Autodesk Inventor part; units mm, degrees
ref_plane "YZ Plane" through (0, 0, 0) normal (1, 0, 0) x (0, 1, 0)
ref_plane "XZ Plane" through (0, 0, 0) normal (0, 1, 0) x (-1, 0, 0)
ref_plane "XY Plane" through (0, 0, 0) normal (0, 0, 1) x (1, 0, 0)
sketch "草图7" plane through (0, 0, 0) normal (0, 1, 0) x (-1, 0, 0)
  line L0 (125, 235) -> (-125, 235)
  line L1 (-125, 235) -> (-125, -235)
  line L2 (-125, -235) -> (125, -235)
  line L3 (125, -235) -> (125, 235)
  line L4 (0, 3) -> (0, -5)
  line L5 (3.5058, 0) -> (-3.4421, 0)
  line L6 (25, 144) -> (-32, 144)
  line L7 (-32, 144) -> (-32, 87)
  line L8 (-32, 87) -> (25, 87)
  line L9 (25, 87) -> (25, 144)
  line L10 (25, 67) -> (-32, 67)
  line L11 (-32, 67) -> (-32, 10)
  line L12 (-32, 10) -> (25, 10)
  line L13 (25, 10) -> (25, 67)
  line L14 (25, -10) -> (-32, -10)
  line L15 (-32, -10) -> (-32, -67)
  line L16 (-32, -67) -> (25, -67)
  line L17 (25, -67) -> (25, -10)
  line L18 (25, -87) -> (-32, -87)
  line L19 (-32, -87) -> (-32, -144)
  line L20 (-32, -144) -> (25, -144)
  line L21 (25, -144) -> (25, -87)
  line L22 (-66, 100) -> (-95, 100)
  line L23 (-95, 100) -> (-95, 54)
  line L24 (-95, 54) -> (-66, 54)
  line L25 (-66, 54) -> (-66, 100)
  line L26 (-66, -54) -> (-95, -54)
  line L27 (-95, -54) -> (-95, -100)
  line L28 (-95, -100) -> (-66, -100)
  line L29 (-66, -100) -> (-66, -54)
  line L30 (100, 15) -> (70, 15)
  line L31 (70, 15) -> (70, -15)
  line L32 (70, -15) -> (100, -15)
  line L33 (100, -15) -> (100, 15)
  circle A0 centre (65, 182) radius 10
  circle A1 centre (65, -182) radius 10
  circle A2 centre (65, 182) radius 15
  circle A3 centre (80, 182) radius 1.5
  circle A4 centre (57.5, 194.9904) radius 1.5
  circle A5 centre (57.5, 169.0096) radius 1.5
  line L34 (125, 235) -> (0, 235)
  line L35 (0, 235) -> (0, 0)
  line L36 (0, 0) -> (125, 0)
  line L37 (125, 0) -> (125, 235)
  line L38 (-125, 235) -> (0, 235)
  line L39 (0, 235) -> (0, 0)
  line L40 (0, 0) -> (-125, 0)
  line L41 (-125, 0) -> (-125, 235)
  line L42 (-125, -235) -> (0, -235)
  line L43 (0, -235) -> (0, 0)
  line L44 (0, 0) -> (-125, 0)
  line L45 (-125, 0) -> (-125, -235)
  line L46 (125, -235) -> (0, -235)
  line L47 (0, -235) -> (0, 0)
  line L48 (0, 0) -> (125, 0)
  line L49 (125, 0) -> (125, -235)
  circle A6 centre (65, -182) radius 15
  circle A7 centre (80, -182) radius 1.5
  circle A8 centre (57.5, -169.0096) radius 1.5
  circle A9 centre (57.5, -194.9904) radius 1.5
  point P0 (0, -87)
  point P1 (0, -67)
  point P2 (0, -10)
  point P3 (0, -235)
  point P4 (0, -144)
  dimension "d115" = 30
  dimension "d118" = 30
  dimension "d84" = 470
  dimension "d85" = 250
  dimension "d86" = 57
  dimension "d87" = 57
  dimension "d88" = 57
  dimension "d89" = 57
  dimension "d90" = 57
  dimension "d91" = 57
  dimension "d92" = 57
  dimension "d93" = 57
  dimension "d94" = 91
  dimension "d95" = 20
  dimension "d96" = 20
  dimension "d97" = 20
  dimension "d98" = 93
  dimension "d99" = 29
  dimension "d100" = 46
  dimension "d101" = 46
  dimension "d102" = 135
  dimension "d103" = 108
  dimension "d104" = 30
  dimension "d105" = 30
  dimension "d106" = 30
  dimension "d107" = 25
  dimension "d108" = 220
  dimension "d109" = 20
  dimension "d110" = 53
  dimension "d111" = 60
  dimension "d112" = 20
  dimension "d113" = 53
  dimension "d114" = 60
  dimension "d116" = 3
  dimension "d117" = 360
  dimension "d119" = 3
  dimension "d120" = 360
extrude "拉伸7" add sketch "草图7" along normal blind 10 contours L40 L5 L4 L43 L14 L15 L16 L18 L19 L20 L2 L1
sketch "草图8" plane through (0, 0, 0) normal (0, -1, 0) x (1, 0, 0)
  line L0 (0, 0) -> (125, 0)
  line L1 (0, -235) -> (0, -144)
  line L2 (47, 0) -> (0, 0)
  line L3 (0, 0) -> (0, -159)
  line L4 (0, -159) -> (47, -159)
  line L5 (47, -159) -> (47, 0)
  line L6 (32, -67) -> (32, -10)
  line L7 (0, -144) -> (32, -144)
  line L8 (111, -39) -> (47, -39)
  line L9 (47, -39) -> (47, -115)
  line L10 (47, -115) -> (111, -115)
  line L11 (111, -115) -> (111, -39)
  line L12 (95, -54) -> (66, -54)
  line L13 (66, -100) -> (95, -100)
  line L14 (95, -100) -> (95, -54)
  line L15 (66, -54) -> (66, -100)
  dimension "d123" = 15
  dimension "d124" = 15
  dimension "d125" = 15
  dimension "d126" = 15
  dimension "d127" = 16
  dimension "d128" = 19
extrude "拉伸8" cut sketch "草图8" against normal blind 5
sketch "草图9" plane through (0, 0, 0) normal (0, -1, 0) x (1, 0, 0)
  line L0 (125, -235) -> (0, -235)
  line L1 (125, 0) -> (111, 0)
  line L2 (111, 0) -> (111, -235)
  line L3 (111, -235) -> (125, -235)
  line L4 (125, -235) -> (125, 0)
  line L5 (0, -235) -> (0, -159)
  line L6 (125, 0) -> (125, -235)
  line L7 (0, -235) -> (125, -235)
  line L8 (125, -235) -> (125, -221)
  line L9 (125, -221) -> (0, -221)
  line L10 (0, -221) -> (0, -235)
  point P0 (0, 0)
  point P1 (111, -221)
  dimension "d131" = 14
  dimension "d132" = 14
extrude "拉伸9" add sketch "草图9" along normal blind 70
sketch "草图10" plane through (0, 10, 0) normal (0, 1, 0) x (1, 0, 0)
  line L0 (0, 221) -> (0, 159)
  line L1 (125, 235) -> (0, 235)
  line L2 (0, 159) -> (10, 159)
  line L3 (10, 159) -> (10, 235)
  line L4 (10, 235) -> (0, 235)
  line L5 (0, 235) -> (0, 159)
  point P0 (0, 0)
  dimension "d135" = 10
extrude "拉伸10" cut sketch "草图10" against normal blind 5
sketch "草图11" plane through (0, 5, 0) normal (0, 1, 0) x (1, 0, 0)
  circle A0 centre (4, 179) radius 2.1
  circle A1 centre (4, 205) radius 2.1
  line L0 (0, 159) -> (0, 235)
  line L1 (10, 159) -> (0, 159)
  line L2 (125, 235) -> (10, 235)
  point P0 (0, 0)
  dimension "d138" = 4.2
  dimension "d139" = 4.2
  dimension "d140" = 4
  dimension "d141" = 4
  dimension "d142" = 20
  dimension "d143" = 30
extrude "拉伸11" cut sketch "草图11" against normal blind 5
sketch "草图12" plane through (125, -70, -235) normal (0, 0, -1) x (-1, 0, 0)
  line L0 (125, 0) -> (125, 75)
  line L1 (14, 0) -> (125, 0)
  line L2 (125, 75) -> (115, 75)
  line L3 (115, 75) -> (115, 0)
  line L4 (115, 0) -> (125, 0)
  line L5 (125, 0) -> (125, 75)
  point P0 (125, 70)
  dimension "d146" = 10
extrude "拉伸12" cut sketch "草图12" against normal blind 7
sketch "草图13" plane through (125, -70, -228) normal (0, 0, -1) x (-1, 0, 0)
  circle A0 centre (121, 50) radius 2.1
  circle A1 centre (121, 20) radius 2.1
  line L0 (125, 75) -> (125, 0)
  line L1 (115, 0) -> (0, 0)
  line L2 (0, 80) -> (115, 80)
  point P0 (125, 70)
  dimension "d149" = 4.2
  dimension "d150" = 4.2
  dimension "d151" = 4
  dimension "d152" = 4
  dimension "d153" = 20
  dimension "d154" = 30
extrude "拉伸13" cut sketch "草图13" against normal blind 7
fillet "圆角2" radius 10 4 edges at (111, 0, -19.5) (111, 0, -168) (55.5, 0, -221) (111, -35, -221)
sketch "草图14" plane through (0, 0, 0) normal (0, -1, 0) x (1, 0, 0)
  circle A0 centre (65, -175) radius 10
  line L0 (125, -235) -> (125, 0)
  line L1 (10, -235) -> (125, -235)
  point P0 (0, 0)
  point P1 (125, -230)
  point P2 (120, -235)
  dimension "d159" = 20
  dimension "d160" = 60
  dimension "d161" = 60
extrude "拉伸14" add sketch "草图14" along normal blind 70
fillet "圆角3" radius 10 1 edges at (55, 0, -175)
sketch "草图16" plane through (0, 10, 0) normal (0, 1, 0) x (1, 0, 0)
  line L0 (125, 0) -> (125, 235)
  line L1 (0, 0) -> (125, 0)
  line L2 (125, 0) -> (125, 10)
  line L3 (125, 10) -> (0, 10)
  line L4 (0, 10) -> (0, 0)
  dimension "d167" = 10
extrude "拉伸16" cut sketch "草图16" against normal blind 5
sketch "草图17" plane through (0, 5, 0) normal (0, 1, 0) x (1, 0, 0)
  circle A0 centre (62, 4) radius 2.1
  circle A1 centre (95, 4) radius 2.1
  line L0 (125, 0) -> (47, 0)
  line L1 (32, 67) -> (32, 10)
  line L2 (125, 10) -> (125, 235)
  point P0 (0, 0)
  dimension "d170" = 4.2
  dimension "d171" = 4.2
  dimension "d172" = 4
  dimension "d173" = 4
  dimension "d174" = 30
  dimension "d175" = 30
extrude "拉伸17" cut sketch "草图17" against normal blind 5
sketch "草图18" plane through (125, -70, -235) normal (1, 0, 0) x (0, 0, -1)
  line L0 (-235, 60) -> (-235, 0)
  line L1 (-225, 75) -> (-235, 75)
  line L2 (-235, 75) -> (-235, 0)
  line L3 (-235, 0) -> (-225, 0)
  line L4 (-225, 0) -> (-225, 75)
  point P0 (-235, 70)
extrude "拉伸18" cut sketch "草图18" against normal blind 7
sketch "草图19" plane through (118, -70, -235) normal (1, 0, 0) x (0, 0, -1)
  circle A0 centre (-231, 50) radius 2.1
  circle A1 centre (-231, 20) radius 2.1
  line L0 (-235, 0) -> (-235, 75)
  line L1 (0, 0) -> (-225, 0)
  line L2 (-225, 80) -> (0, 80)
  point P0 (-235, 70)
  dimension "d180" = 4.2
  dimension "d181" = 4.2
  dimension "d182" = 4
  dimension "d183" = 4
  dimension "d184" = 20
  dimension "d185" = 30
extrude "拉伸19" cut sketch "草图19" against normal blind 7
fillet "圆角4" radius 5 3 edges at (125, 10, -122.5) (67.5, 10, -235) (125, -30, -235)
properties part number "top_4"
Model file for the job. Use its own axes, mm. A direction names the side the tool comes from. Coordinates: 2 decimals unless noted, no trailing zeros. Loops run counter-clockwise (first coordinate to the right, second up) from the corner with the lowest first, then second, coordinate; pieces in that order, holes last. Notation, with made-up numbers: (-2, -16) -> (17, -16) arc R10 ccw to (17, 0) -> close; hole circle Ø5 at (17.25, 54.5). An arc over 180 degrees is marked (long way). Use one line per item in the form item = value. Start each with the question number.
(1) Probe probe 1 along X at (y, z) = (2.1, -4); probe 2 along Y at (x, z) = (114.25, -4); probe 3 along Z at (x, y) = (106, 0). List the from-to ranges inside material, lowest first. Write a range as from..to.
(2) Cut at B-B on z = -62. Give the cut face in (x, y).
(3) Flat gauge pins, fed straight in: pin 1 (2 mm diameter, centred on y = -60, z = -41, fed in from -X); pin 2 (1 mm diameter, centred on x = 24, y = -24, fed in from +Z); pin 3 (2.5 mm diameter, centred on y = 1.5, z = -21, fed in from -X); pin 4 (4 mm diameter, centred on y = -20, z = -4, fed in from +X). Where does each tip first touch, or does it go through?
(4) Cut at D-D on z = -199.5. Give the cut face in (x, y), and give its area (3 significant figures).
(5) Pull direction Z, two halves, no side cores. Call faces 6 (the flat face through (125, -33, -118)), 7 (the flat face through (81, 1, -115)), 8 (the flat face through (23, 2, -159)), 9 (the flat face through (16, 7, -87)): pulls with the +Z half, pulls with the -Z half, needs draft (parallel to the pull), parting line crosses it, or undercut.
(6) Tool access for faces 1 (the flat face through (47, 2, -137)), 2 (the flat face through (118, -32, -5)), 3 (the cylindrical face through (107.99, -2.85, -163.67)), 4 (the flat face through (16, 7, -144)), 5 (the flat face through (32, 7, -38)): list every direction of +Z, -Z, +X, -X, +Y, -Y with a clear straight run to the whole face (end or side of a thin tool).
(7) Cut at A-A on y = -55.5. Give the cut face in (x, z).
(8) Cut at C-C on z = -122.5. Give the cut face in (x, y).
Values:
q1.probe_1 = 47..59.9, 64.1..92.9, 97.1..118
q1.probe_2 = -70..-52.1, -47.9..-22.1, -17.9..5
q1.probe_3 = -235..-115, -39..0
q2.outline = (32, 5) -> (66, 5) -> (66, 10) -> (32, 10) -> close; (95, 5) -> (111, 5) -> (111, -70) -> (125, -70) -> (125, 5) arc R5 ccw to (120, 10) -> (95, 10) -> close
q3.pin_1 = 111
q3.pin_2 = -221
q3.pin_3 = 47
q3.pin_4 = through
q4.outline = (0, 0) -> (101, 0) arc R10 cw to (111, -10) -> (111, -70) -> (125, -70) -> (125, 5) arc R5 ccw to (120, 10) -> (10, 10) -> (10, 5) -> (0, 5) -> close
q4.area = 2,200 mm2
q5.face_6 = needs draft
q5.face_7 = undercut
q5.face_8 = pulls with the +Z half
q5.face_9 = undercut
q6.face_1 = +Z, -X, -Y
q6.face_2 = +Z, +X, +Y, -Y
q6.face_3 = +Z, -Y
q6.face_4 = -X, +Y, -Y
q6.face_5 = +Z, -X, +Y, -Y
q7.outline = (0, -228) -> (10, -228) -> (10, -235) -> (120, -235) arc R5 ccw to (125, -230) -> (125, -10) -> (118, -10) -> (118, 0) -> (111, 0) -> (111, -211) arc R10 cw to (101, -221) -> (0, -221) -> close; circle Ø20 at (65, -175)
q8.outline = (32, 5) -> (47, 5) -> (47, 0) -> (101, 0) arc R10 cw to (111, -10) -> (111, -70) -> (125, -70) -> (125, 5) arc R5 ccw to (120, 10) -> (32, 10) -> close
